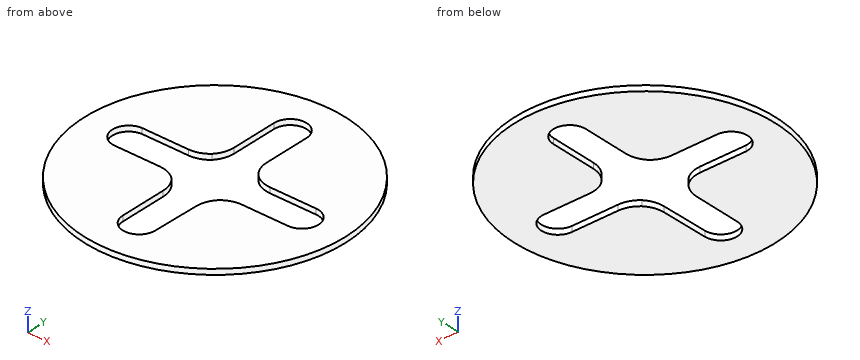
from build123d import *

# Parameters (mm, degrees)
F0_R         = 38.1
F1_DEPTH     = 1.5875
F2_T1_DEPTH  = 19.6594045054
F2_T3_DEPTH  = 19.7689044348
F2_T5_DEPTH  = 19.8002867112
F2_T7_DEPTH  = 19.8028708993
F2_T9_DEPTH  = 19.7937834769
F2_T11_DEPTH = 19.3627357335
F2_T13_DEPTH = 19.2813787557
F2_T15_DEPTH = 19.9326468644


# Not quite as in the source:
# - a fillet or chamfer that OpenCascade refuses, or shapes differently, is made with other operations: its cross-section is extruded or revolved along the edge and cut away or added


with BuildPart() as f1:
    # F0 (on Top) → F1 (new body)
    with BuildSketch(Plane.XY):
        Circle(F0_R)
        with BuildLine():
            ThreePointArc((25.5212023113, 4.7665246553), (30.2837023113, 0.0040246553), (25.5212023113, -4.7584753447))
            Line((25.5212023113, -4.7584753447), (8.3700942824, -4.7584753447))
            ThreePointArc((8.3700942824, -4.7584753447), (6.8307613912, -6.7854450641), (4.8140826203, -8.3382356902))
            Line((4.8140826203, -8.3382356902), (4.5445678914, -25.4872259938))
            ThreePointArc((4.5445678914, -25.4872259938), (-0.2648058004, -30.1554173191), (-4.9795027497, -25.3916248979))
            Line((-4.9795027497, -25.3916248979), (-4.9795027497, -8.2405168689))
            ThreePointArc((-4.9795027497, -8.2405168689), (-6.9221674375, -6.692171835), (-8.4040103572, -4.6983162748))
            Line((-8.4040103572, -4.6983162748), (-25.5551183861, -4.6983162748))
            ThreePointArc((-25.5551183861, -4.6983162748), (-30.0672979191, 0.0912532901), (-25.4878952685, 4.8165905393))
            Line((-25.4878952685, 4.8165905393), (-8.3367872396, 4.8165905393))
            ThreePointArc((-8.3367872396, 4.8165905393), (-6.7888119889, 6.8274151536), (-4.7692424862, 8.3639638934))
            Line((-4.7692424862, 8.3639638934), (-4.7692424862, 25.5150719223))
            ThreePointArc((-4.7692424862, 25.5150719223), (-0.0106390137, 30.260270074), (4.7556603142, 25.5228020557))
            Line((4.7556603142, 25.5228020557), (4.7556603142, 8.3716940268))
            ThreePointArc((4.7556603142, 8.3716940268), (6.8069974407, 6.8092842314), (8.3700961728, 4.7584720195))
            Line((8.3700961728, 4.7584720195), (25.5212023113, 4.7665246553))
        make_face(mode=Mode.SUBTRACT)
    extrude(amount=F1_DEPTH)

    # F2: fillet of radius 7.62 on 8 edges, made by hand

    # F2_s2 → F2_t1 (cut)
    with BuildSketch(Plane.XY.offset(-9.0359522527)):
        with BuildLine():
            ThreePointArc((-11.9511681406, 4.8165905393), (-9.1053172731, 5.3679603439), (-6.6713079375, 6.9422774581))
            ThreePointArc((-6.6713079375, 6.9422774581), (-7.5789423028, 5.9381141343), (-8.3367872396, 4.8165905393))
            Line((-8.3367872396, 4.8165905393), (-11.9511681406, 4.8165905393))
        make_face()
    extrude(amount=F2_T1_DEPTH, mode=Mode.SUBTRACT)

    # F2_s4 → F2_t3 (cut)
    with BuildSketch(Plane.XY.offset(-9.0907022174)):
        with BuildLine():
            ThreePointArc((-6.9158471176, 6.6987031989), (-5.3262518764, 9.1404259669), (-4.7692424862, 12.0002447803))
            Line((-4.7692424862, 12.0002447803), (-4.7692424862, 8.3639638934))
            ThreePointArc((-4.7692424862, 8.3639638934), (-5.9015763197, 7.607428136), (-6.9158471176, 6.6987031989))
        make_face()
    extrude(amount=F2_T3_DEPTH, mode=Mode.SUBTRACT)

    # F2_s6 → F2_t5 (cut)
    with BuildSketch(Plane.XY.offset(-9.1063933556)):
        with BuildLine():
            ThreePointArc((4.7556603142, 12.014251369), (5.3142882964, 9.1504383117), (6.9082653607, 6.7065218711))
            ThreePointArc((6.9082653607, 6.7065218711), (5.8910941356, 7.615548292), (4.7556603142, 8.3716940268))
            Line((4.7556603142, 8.3716940268), (4.7556603142, 12.014251369))
        make_face()
    extrude(amount=F2_T5_DEPTH, mode=Mode.SUBTRACT)

    # F2_s8 → F2_t7 (cut)
    with BuildSketch(Plane.XY.offset(-9.1076854497)):
        with BuildLine():
            ThreePointArc((6.703921101, 6.9107892294), (9.1487661341, 5.3175989867), (12.0131699511, 4.7601824833))
            Line((12.0131699511, 4.7601824833), (8.3700961728, 4.7584720195))
            ThreePointArc((8.3700961728, 4.7584720195), (7.6134497132, 5.893806017), (6.703921101, 6.9107892294))
        make_face()
    extrude(amount=F2_T7_DEPTH, mode=Mode.SUBTRACT)

    # F2_s10 → F2_t9 (cut)
    with BuildSketch(Plane.XY.offset(-9.1031417385)):
        with BuildLine():
            ThreePointArc((12.0113509777, -4.7584753447), (9.1483653066, -5.3167678283), (6.7049028325, -6.9098367498))
            ThreePointArc((6.7049028325, -6.9098367498), (7.6138671828, -5.8932667023), (8.3700942824, -4.7584753447))
            Line((8.3700942824, -4.7584753447), (12.0113509777, -4.7584753447))
        make_face()
    extrude(amount=F2_T9_DEPTH, mode=Mode.SUBTRACT)

    # F2_s12 → F2_t11 (cut)
    with BuildSketch(Plane.XY.offset(-8.8876178667)):
        with BuildLine():
            ThreePointArc((6.90916797, -6.7055919846), (5.3384286521, -9.0938512154), (4.7582181499, -11.8928438791))
            Line((4.7582181499, -11.8928438791), (4.8140826203, -8.3382356902))
            ThreePointArc((4.8140826203, -8.3382356902), (5.9181950346, -7.5945067933), (6.90916797, -6.7055919846))
        make_face()
    extrude(amount=F2_T11_DEPTH, mode=Mode.SUBTRACT)

    # F2_s14 → F2_t13 (cut)
    with BuildSketch(Plane.XY.offset(-8.8469393778)):
        with BuildLine():
            ThreePointArc((-4.9795027497, -11.7792926201), (-5.5115025024, -8.9820345887), (-7.0332173151, -6.5753646363))
            ThreePointArc((-7.0332173151, -6.5753646363), (-6.06378956, -7.478771428), (-4.9795027497, -8.2405168689))
            Line((-4.9795027497, -8.2405168689), (-4.9795027497, -11.7792926201))
        make_face()
    extrude(amount=F2_T13_DEPTH, mode=Mode.SUBTRACT)

    # F2_s16 → F2_t15 (cut)
    with BuildSketch(Plane.XY.offset(-9.1725734322)):
        with BuildLine():
            ThreePointArc((-6.7393383503, -6.8762551219), (-9.1924239959, -5.2637820597), (-12.0730397301, -4.6983162748))
            Line((-12.0730397301, -4.6983162748), (-8.4040103572, -4.6983162748))
            ThreePointArc((-8.4040103572, -4.6983162748), (-7.6495821405, -5.8468332435), (-6.7393383503, -6.8762551219))
        make_face()
    extrude(amount=F2_T15_DEPTH, mode=Mode.SUBTRACT)


solid = f1.part
Check sheet for the modelled part. Datum: model origin and axes. Units: mm. Round coordinates to 2 decimals unless told otherwise and drop trailing zeros. Loops run counter-clockwise (first coordinate to the right, second up) from the corner with the lowest first, then second, coordinate; pieces in that order, holes last. Notation, with made-up numbers: (-31.5, 63.5) -> (24.5, 63.5) arc R21 cw to (24.5, 92.5) -> close; hole circle Ø7 at (-31.75, 47.5). An arc over 180 degrees is marked (long way). Put each result on its own line as item: value. Start each with the question number.
1. Section check C-C (z = 0.8). Enter the section's corners in (x, y) (1 decimal).
2. Section check B-B (y = 23). Enter the section's corners in (x, z), plus the area to 3 significant figures.
3. Gauge pin test, flat ends, axial feed: pin 1 (0.8 mm diameter, centred on y = -16.5, z = 1, fed in from +X); pin 2 (0.8 mm diameter, centred on y = 22, z = 0.5, fed in from -X). Record the tip position at first contact, or that the pin passes through.
4. Scan lines: probe 1 along X at (y, z) = (-18.5, 0.25); probe 2 along X at (y, z) = (-3, 0.8); probe 3 along Y at (x, z) = (-1, 0.85). Record each from-to range of solid material in increasing order.
5. Section check D-D (x = -31). Enter the section's corners in (y, z).
6. Section check A-A (x = 23). Enter the section's corners in (y, z).
Findings:
1. outline: circle Ø76.2 at (0, 0); hole (-25.6, -4.7) -> (-12.1, -4.7) arc R7.6 cw to (-6.9, -6.7) arc R7.6 cw to (-5, -11.8) -> (-5, -25.4) arc R4.8 ccw to (4.5, -25.5) -> (4.8, -11.9) arc R7.6 cw to (6.8, -6.8) arc R7.6 cw to (12, -4.8) -> (25.5, -4.8) arc R4.8 ccw to (25.5, 4.8) -> (12, 4.8) arc R7.6 cw to (6.8, 6.8) arc R7.6 cw to (4.8, 12) -> (4.8, 25.5) arc R4.8 ccw to (-4.8, 25.5) -> (-4.8, 12) arc R7.6 cw to (-6.8, 6.8) arc R7.6 cw to (-12, 4.8) -> (-25.5, 4.8) arc R4.8 ccw to start
2. outline: (-30.37, 0) -> (-4.77, 0) -> (-4.77, 1.59) -> (-30.37, 1.59) -> close; (4.76, 0) -> (30.37, 0) -> (30.37, 1.59) -> (4.76, 1.59) -> close
2. area: 81.3 mm^2
3. pin 1: stops at x = 34.53
3. pin 2: stops at x = -31.39
4. probe 1: x = -33.31 to -4.98, 4.65 to 33.31
4. probe 2: x = -37.98 to -28.96, 29.22 to 37.98
4. probe 3: y = -38.09 to -30.09, 30.16 to 38.09
5. outline: (-22.15, 0) -> (22.15, 0) -> (22.15, 1.59) -> (-22.15, 1.59) -> close
6. outline: (-30.37, 0) -> (-4.76, 0) -> (-4.76, 1.59) -> (-30.37, 1.59) -> close; (4.77, 0) -> (30.37, 0) -> (30.37, 1.59) -> (4.77, 1.59) -> close
